Job drawing, mm, ordinate dimensions from the low corner. One solid piece. A direction names the side the tool comes from. Round coordinates to 2 decimals unless told otherwise and drop trailing zeros. Write each loop counter-clockwise with the first axis right and the second up, starting at its lowest first coordinate (ties: lowest second). Pieces come first, ordered by that corner, then holes.
1) Wall check: probe 1 along Z at (x, y) = (2.5, 6.75) (1 decimal); probe 2 along X at (y, z) = (5, 15) (1 decimal); probe 3 along Y at (x, z) = (9.5, 9). Give the ranges that are in metal, low to high.
2) Which spindle directions (+Z, -Z, +X, -X, +Y, -Y) get a long thin tool onto all of the face, cutting with end or side? Do the marked faces 1 and 2. Say none if no direction does.
3) Saw through at A-A (z = 19). Write the cut outline in (x, y) (1 decimal).
4) Saw through at B-B (x = 15.5). Write the cut outline in (y, z) (1 decimal).
5) Flat gauge pins, fed straight in: pin 1 (3 mm diameter, centred on y = 7, z = 5.5, fed in from +X); pin 2 (6 mm diameter, centred on x = 1.5, z = 23, fed in from -Y) (1 decimal); pin 3 (1.5 mm diameter, centred on x = 3, y = 11, fed in from -Z). Where does each tip first touch, or does it go through?
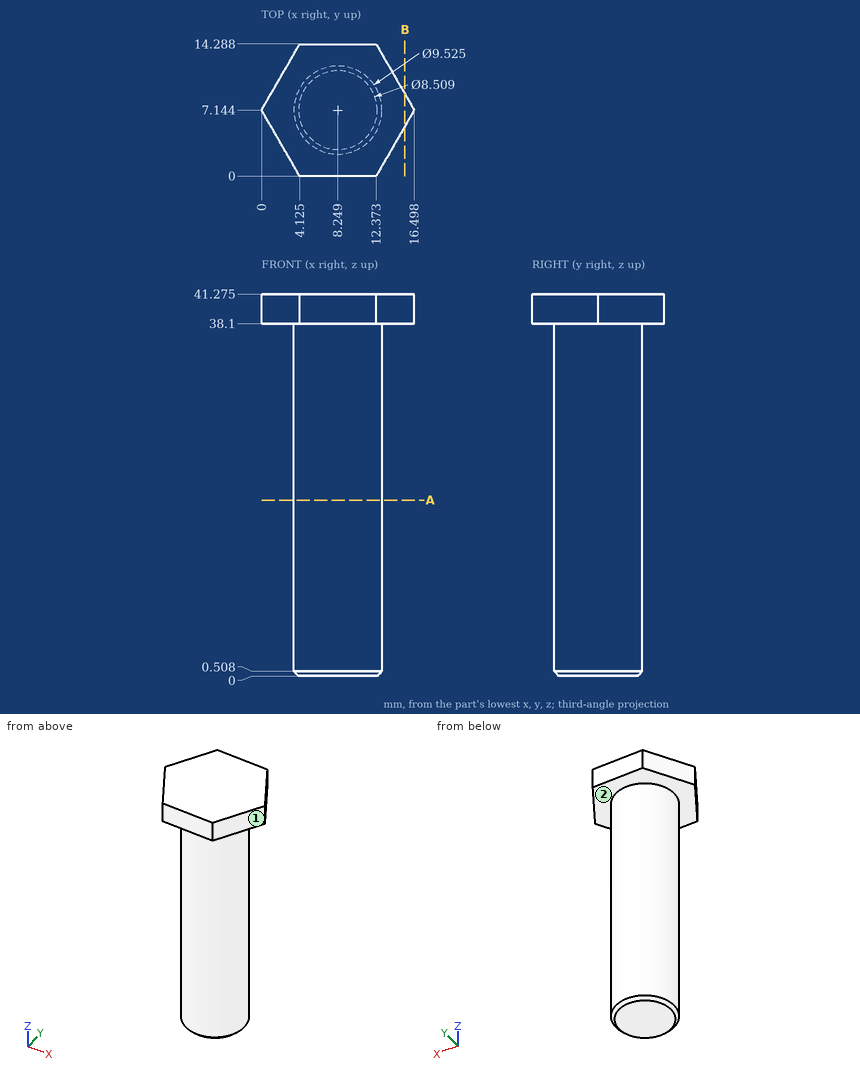
Evaluation:
1. probe 1: z = 38.1 to 41.3
1. probe 2: x = 4 to 12.5
1. probe 3: y = 2.55 to 11.74
2. face 1: +Z, -Z, +X, -Y
2. face 2: -Z
3. outline: circle Ø9.5 at (8.2, 7.1)
4. outline: (5.4, 38.1) - (8.9, 38.1) - (8.9, 41.3) - (5.4, 41.3) - close
5. pin 1: stops at x = 13.01
5. pin 2: stops at y = 4.2
5. pin 3: stops at z = 38.1
